Drawing for the job (mm, zero at the part's lowest x, y, z). A direction names the side the tool comes from. Give positions to 0.01 mm unless a question says otherwise; leave off trailing zeros. Write each loop counter-clockwise with the first axis right and the second up, starting at its lowest first coordinate (ties: lowest second). Pieces come first, ordered by that corner, then holes. Notation, with made-up numbers: M -5.75,-26.5 L 34.25,-26.5 A21 ccw 34.25,-14.5 Z; hole C 33,3 d6. An arc over 180 degrees is marked long. Use CSV: the item, a comma, the result in double quotes. Start each with the question number.
1. Mould opens along X. For the marked faces 1, 2 and 3 say: pulls with the +X half, pulls with the -X half, needs draft (parallel to the pull), parting line crosses it, or undercut.
2. Band-saw the part on B-B, the plane x = 12.1. List the corners of the cut face in (y, z).
3. Band-saw the part on A-A, the plane z = 7.9. List the corners of the cut face in (x, y).
4. Band-saw the part on D-D, the plane z = 6. List the corners of the cut face in (x, y), then the cut area to 3 significant figures.
5. Drop flat-ended pins along their axis: pin 1 Ø3.5 at (x, z) = (12.1, 7.9) entering from +Y; pin 2 Ø5 at (x, y) = (12, 5.5) entering from -Z. Give the stop position or say it passes through.
6. Band-saw the part on C-C, the plane y = 2.75. List the corners of the cut face in (x, z), then the cut area to 3 significant figures.
7. Drill centre lines: line 1 along X through (y, z) = (11.45, 7.9); line 2 along Y through (x, z) = (15.25, 7.5); line 3 along Z through (x, y) = (13.5, 7.5). Where is each one in solid material? Low to high. Write a range as from..to.
8. 3-axis set-ups, long thin cutter, end or side, ignore diameter. For the marked faces 4 and 5: which of +Z, -Z, +X, -X, +Y, -Y reach the whole face in a straight line?
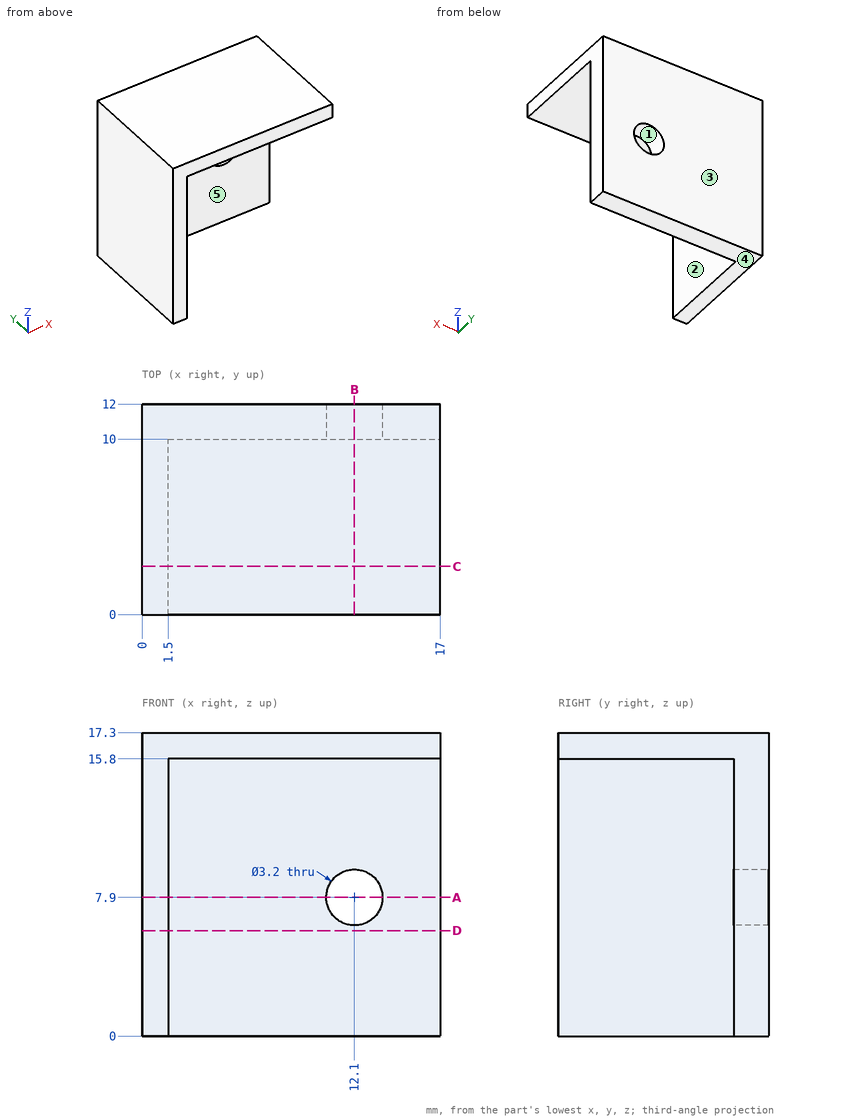
Output:
1,face 1,"undercut"
1,face 2,"pulls with the +X half"
1,face 3,"needs draft"
2,outline,"M 0,15.8 L 10,15.8 L 10,9.5 L 12,9.5 L 12,17.3 L 0,17.3 Z; M 10,0 L 12,0 L 12,6.3 L 10,6.3 Z"
3,outline,"M 0,0 L 1.5,0 L 1.5,10 L 10.5,10 L 10.5,12 L 0,12 Z; M 13.7,10 L 17,10 L 17,12 L 13.7,12 Z"
4,outline,"M 0,0 L 1.5,0 L 1.5,10 L 17,10 L 17,12 L 0,12 Z"
4,area,"49.0 mm²"
5,pin 1,"stops at y = 12"
5,pin 2,"stops at z = 15.8"
6,outline,"M 0,0 L 1.5,0 L 1.5,15.8 L 17,15.8 L 17,17.3 L 0,17.3 Z"
6,area,"49.2 mm²"
7,line 1,"x = 0..10.5, 13.7..17"
7,line 2,"y = 10..12"
7,line 3,"z = 15.8..17.3"
8,face 4,"-Z, +X, -X, +Y, -Y"
8,face 5,"-Z, +X, -Y"
